Build history of the part. All positions in model axes, mm. Face numbers are marked on the shaded views. A direction names the side the tool comes from. Round coordinates to 2 decimals unless told otherwise and drop trailing zeros. Write each loop counter-clockwise with the first axis right and the second up, starting at its lowest first coordinate (ties: lowest second). Pieces come first, ordered by that corner, then holes.
Item 1: Drop flat-ended pins along their axis: pin 1 Ø5 at (x, z) = (36.5, -12) entering from +Y; pin 2 Ø1 at (x, z) = (24, -6.5) entering from +Y; pin 3 Ø2.5 at (x, z) = (33, 4) entering from +Y. Give the stop position or say it passes through.
Item 2: 3-axis set-ups, long thin cutter, end or side, ignore diameter. For the marked faces 1 and 2: which of +Z, -Z, +X, -X, +Y, -Y reach the whole face in a straight line?
Item 3: Band-saw the part on B-B, the plane y = 0. Count the separate pieces of the cut face and the enclosed holes in it, then the cut area to 3 significant figures.
Item 4: Band-saw the part on A-A, the plane y = -7.25. Write the cut outline in (x, z).
Item 5: Mould opens along Z. For the marked faces 3, 4 and 5 say: +Z half, -Z half, draft (parallel to the pull), parting line (faces both ways), or undercut.
Item 6: Wall check: probe 1 along X at (y, z) = (-5.25, 0); probe 2 along Z at (x, y) = (25, 2.25); probe 3 along X at (y, z) = (-12.7, 0.05). Give the ranges that are in metal, low to high.
```python
from build123d import *
from OCP.BRepFilletAPI import BRepFilletAPI_MakeFillet

# Parameters (mm, degrees)
BOSS_EXTRUDE1_DEPTH       = 45.72
CUT_EXTRUDE1_DEPTH        = 59.101632507
FILLET2_R                 = 16.51
FILLET3_R                 = 16.51
SKETCH3_OUTSIDE_W         = 60.308
SKETCH3_OUTSIDE_H         = 47.608
CUT_EXTRUDE2_DEPTH        = 52.759317573
SKETCH5_W                 = 24.000000006
SKETCH5_H                 = 12.5
CUT_EXTRUDE3_DEPTH        = 8.16
CUT_EXTRUDE4_DEPTH        = 56.097932423
FILLET4_R1                = 3
FILLET4_R2                = 5
F_2_0MM_DOWEL_HOLE1_D     = 2
F_2_0MM_DOWEL_HOLE1_DEPTH = 8
F_2_0MM_DOWEL_HOLE1_TIP   = 0.600860619
SKETCH11_R                = 2.5
SKETCH11_R_2              = 1.3
CUT_EXTRUDE6_DEPTH        = 5.08
CUT_EXTRUDE7_DEPTH        = 1.5


with BuildPart() as part:
    # Sketch1 → Boss-Extrude1 (new body)
    with BuildSketch(Plane.YZ):
        with BuildLine():
            Line((10.668, -16.51), (-10.668, -16.51))
            ThreePointArc((-10.668, -16.51), (-13.002866591, -15.542866591), (-13.97, -13.208))
            Line((-13.97, -13.208), (-13.97, 13.208))
            ThreePointArc((-13.97, 13.208), (-13.002866591, 15.542866591), (-10.668, 16.51))
            Line((-10.668, 16.51), (10.668, 16.51))
            ThreePointArc((10.668, 16.51), (13.002866591, 15.542866591), (13.97, 13.208))
            Line((13.97, 13.208), (13.97, -13.208))
            ThreePointArc((13.97, -13.208), (13.002866591, -15.542866591), (10.668, -16.51))
        make_face()
    extrude(amount=BOSS_EXTRUDE1_DEPTH)

    # Sketch2 → Cut-Extrude1 (cut, through all)
    with BuildSketch(Plane(origin=(0, 0, -16.51), x_dir=(1, 0, 0), z_dir=(0, 0, -1))):
        with BuildLine():
            Line((5.08, -13.97), (45.72, -13.97))
            Line((45.72, -13.97), (45.72, 4.03))
            add(Edge.make_bspline(
                [(5.08, -13.97), (23.327246471, -0.48405524), (45.72, 4.03)],
                knots=[0, 0, 0, 1, 1, 1], degree=2))
        make_face()
    extrude(amount=-CUT_EXTRUDE1_DEPTH, mode=Mode.SUBTRACT)

    # Fillet2
    # the kernel refuses this fillet: 16.51 mm, written as the material it takes off along each edge
    with BuildSketch(Plane(origin=(45.72, 37.245, -16.51), x_dir=(-1, 0, 0), z_dir=(0, -1, 0))) as fillet2_piece_1:
        with BuildLine():
            CenterArc((FILLET2_R, -FILLET2_R), FILLET2_R, 90, 90)
            Line((0, -FILLET2_R), (0, 0))
            Line((0, 0), (FILLET2_R, 0))
        make_face()
    extrude(amount=89.188, mode=Mode.SUBTRACT)

    # Fillet3
    # the kernel refuses this fillet: 16.51 mm, written as the material it takes off along each edge
    with BuildSketch(Plane(origin=(45.72, -51.943, 16.51), x_dir=(-1, 0, 0), z_dir=(0, 1, 0))) as fillet3_piece_1:
        with BuildLine():
            CenterArc((FILLET3_R, -FILLET3_R), FILLET3_R, 90, 90)
            Line((0, -FILLET3_R), (0, 0))
            Line((0, 0), (FILLET3_R, 0))
        make_face()
    extrude(amount=89.188, mode=Mode.SUBTRACT)

    # Sketch3 outside → Cut-Extrude2 (cut, through all)
    # profile 1 of 2: a face of its own
    with BuildSketch(Plane(origin=(0, -3.81, 0), x_dir=(-1, 0, 0), z_dir=(0, -1, 0))):
        with Locations((-22.86, 0)):
            Rectangle(SKETCH3_OUTSIDE_W, SKETCH3_OUTSIDE_H)
        with BuildLine():
            Line((-29.21, -16.51), (0, -16.51))
            Line((0, -16.51), (0, 16.51))
            Line((0, 16.51), (-29.21, 16.51))
            ThreePointArc((-29.21, 16.51), (-45.72, 0), (-29.21, -16.51))
        make_face(mode=Mode.SUBTRACT)
    # profile 2 of 2: a face of its own
    with BuildSketch(Plane(origin=(0, -3.81, 0), x_dir=(-1, 0, 0), z_dir=(0, -1, 0))):
        with BuildLine():
            Line((-29.21, -13.97), (-5.08, -13.97))
            Line((-5.08, -13.97), (-5.08, 13.97))
            Line((-5.08, 13.97), (-29.21, 13.97))
            ThreePointArc((-29.21, 13.97), (-43.18, 0), (-29.21, -13.97))
        make_face()
    extrude(amount=-CUT_EXTRUDE2_DEPTH, mode=Mode.SUBTRACT)

    # Sketch5 → Cut-Extrude3 (cut)
    with BuildSketch(Plane(origin=(0, -3.81, 0), x_dir=(-1, 0, 0), z_dir=(0, -1, 0))):
        with Locations((-24.080000003, 0)):
            Rectangle(SKETCH5_W, SKETCH5_H)
    extrude(amount=CUT_EXTRUDE3_DEPTH, mode=Mode.SUBTRACT)

    # Sketch6 → Cut-Extrude4 (cut, through all)
    with BuildSketch(Plane(origin=(0, -11.97, 0), x_dir=(-1, 0, 0), z_dir=(0, 1, 0))):
        with BuildLine():
            ThreePointArc((-24.267500006, 3.099974385), (-36.080000006, 0.05), (-24.267500006, -2.999974385))
            ThreePointArc((-24.267500006, -2.999974385), (-20.330000006, 0.05), (-24.267500006, 3.099974385))
        make_face()
    extrude(amount=-CUT_EXTRUDE4_DEPTH, mode=Mode.SUBTRACT)

    # Fillet4: one fillet with a radius per group of edges: ONE call of the kernel's fillet builder (fillet() takes one radius for all edges)
    fillet4_edges_1 = [part.edges().sort_by_distance(p)[0] for p in [
        (24.267500006, -12.97, 3.099974385),
    ]]
    fillet4_edges_2 = [part.edges().sort_by_distance(p)[0] for p in [
        (24.267500006, -12.97, -2.999974385),
    ]]
    fillet4 = BRepFilletAPI_MakeFillet(part.part.solid().wrapped)
    for e in fillet4_edges_1:
        fillet4.Add(FILLET4_R1, e.wrapped)
    for e in fillet4_edges_2:
        fillet4.Add(FILLET4_R2, e.wrapped)
    add(Compound.cast(fillet4.Shape()), mode=Mode.REPLACE)

    # Ø2.0mm Dowel Hole1
    with Locations(Plane(origin=(0, -3.81, 0), x_dir=(-1, 0, 0), z_dir=(0, 1, 0))):
        with Locations((-10.08, 0), (-38.080000006, 0)):
            Hole(F_2_0MM_DOWEL_HOLE1_D / 2, depth=F_2_0MM_DOWEL_HOLE1_DEPTH)
            with Locations((0, 0, -(F_2_0MM_DOWEL_HOLE1_DEPTH + F_2_0MM_DOWEL_HOLE1_TIP / 2))):  # 118° drill point
                Cone(0, F_2_0MM_DOWEL_HOLE1_D / 2, F_2_0MM_DOWEL_HOLE1_TIP, mode=Mode.SUBTRACT)

    # Sketch11 → Cut-Extrude6 (cut)
    with BuildSketch(Plane(origin=(0, 0, 0), x_dir=(0, -1, 0), z_dir=(-1, 0, 0))):
        with Locations(Location((0, -5.08, 0), (0, 0, 90))):
            Circle(SKETCH11_R)
        with Locations(Location((0, -0.58, 0), (0, 0, 90))):
            Circle(SKETCH11_R_2)
        with Locations(Location((0, -9.58, 0), (0, 0, 90))):
            Circle(SKETCH11_R_2)
    extrude(amount=-CUT_EXTRUDE6_DEPTH, mode=Mode.SUBTRACT)

    # Sketch12 → Cut-Extrude7 (cut)
    with BuildSketch(Plane(origin=(0, 0, 0), x_dir=(0, -1, 0), z_dir=(-1, 0, 0))):
        with BuildLine():
            Line((1.3, -9.58), (2.5, -9.58))
            ThreePointArc((2.5, -9.58), (2.118290802, -8.252278614), (1.089724736, -7.33))
            ThreePointArc((1.089724736, -7.33), (0, -7.58), (-1.089724736, -7.33))
            ThreePointArc((-1.089724736, -7.33), (-2.118290802, -8.252278614), (-2.5, -9.58))
            Line((-2.5, -9.58), (-1.3, -9.58))
            ThreePointArc((-1.3, -9.58), (0, -8.28), (1.3, -9.58))
        make_face()
        with BuildLine():
            Line((2.5, -5.08), (2.5, -0.58))
            ThreePointArc((2.5, -0.58), (2.118290802, -1.907721386), (1.089724736, -2.83))
            ThreePointArc((1.089724736, -2.83), (2.118290802, -3.752278614), (2.5, -5.08))
        make_face()
        with BuildLine():
            Line((2.5, -9.58), (2.5, -5.08))
            ThreePointArc((2.5, -5.08), (2.118290802, -6.407721386), (1.089724736, -7.33))
            ThreePointArc((1.089724736, -7.33), (2.118290802, -8.252278614), (2.5, -9.58))
        make_face()
        with BuildLine():
            ThreePointArc((-1.089724736, -7.33), (-2.118290802, -6.407721386), (-2.5, -5.08))
            Line((-2.5, -5.08), (-2.5, -9.58))
            ThreePointArc((-2.5, -9.58), (-2.118290802, -8.252278614), (-1.089724736, -7.33))
        make_face()
        with BuildLine():
            ThreePointArc((-1.089724736, -2.83), (-2.118290802, -1.907721386), (-2.5, -0.58))
            Line((-2.5, -0.58), (-2.5, -5.08))
            ThreePointArc((-2.5, -5.08), (-2.118290802, -3.752278614), (-1.089724736, -2.83))
        make_face()
        with BuildLine():
            ThreePointArc((1.089724736, -2.83), (2.118290802, -1.907721386), (2.5, -0.58))
            Line((2.5, -0.58), (1.3, -0.58))
            ThreePointArc((1.3, -0.58), (0, -1.88), (-1.3, -0.58))
            Line((-1.3, -0.58), (-2.5, -0.58))
            ThreePointArc((-2.5, -0.58), (-2.118290802, -1.907721386), (-1.089724736, -2.83))
            ThreePointArc((-1.089724736, -2.83), (0, -2.58), (1.089724736, -2.83))
        make_face()
        with BuildLine():
            Line((1.3, -0.58), (2.5, -0.58))
            ThreePointArc((2.5, -0.58), (0, 1.92), (-2.5, -0.58))
            Line((-2.5, -0.58), (-1.3, -0.58))
            ThreePointArc((-1.3, -0.58), (0, 0.72), (1.3, -0.58))
        make_face()
        with BuildLine():
            ThreePointArc((-2.5, -9.58), (0, -12.08), (2.5, -9.58))
            Line((2.5, -9.58), (1.3, -9.58))
            ThreePointArc((1.3, -9.58), (0, -10.88), (-1.3, -9.58))
            Line((-1.3, -9.58), (-2.5, -9.58))
        make_face()
    extrude(amount=-CUT_EXTRUDE7_DEPTH, mode=Mode.SUBTRACT)


solid = part.part
```
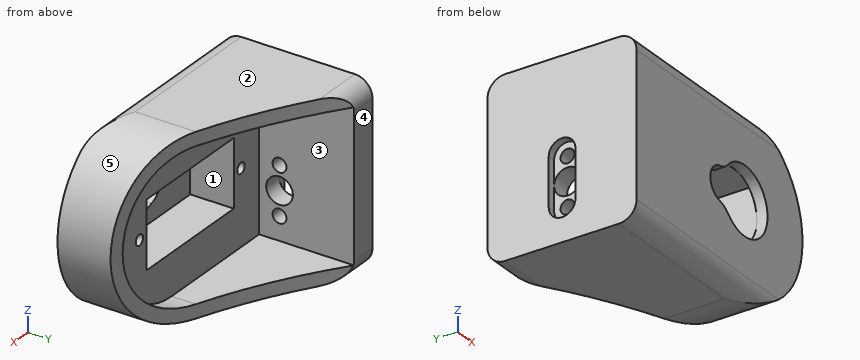
Results:
1. pin 1: stops at y = -1.03
1. pin 2: stops at y = -3.81
1. pin 3: stops at y = -11.97
2. face 1: +Y
2. face 2: +Z, +X, -X, +Y, -Y
3. separate pieces: 4
3. enclosed holes: 0
3. area: 243 mm2
4. outline: (0, -16.51) - (29.21, -16.51) arc R16.51 ccw to (29.21, 16.51) - (0, 16.51) - close; hole circle Ø2 at (10.08, 0); hole (12.08, -6.25) - (36.08, -6.25) - (36.08, 6.25) - (12.08, 6.25) - close; hole circle Ø2 at (38.08, 0)
5. face 3: undercut
5. face 4: draft
5. face 5: parting line
6. probe 1: x = 0 to 9.08, 11.08 to 12.08, 36.08 to 37.08, 39.08 to 45.72
6. probe 2: z = -16.51 to -13.97, 13.97 to 16.51
6. probe 3: x = 0 to 20.33, 36.08 to 45.72
